```python
from build123d import *


with BuildPart() as part:
    # Sketch1 → Revolve1 (revolve)
    with BuildSketch(Plane(origin=(0, 0, 0), x_dir=(1, 0, 0), z_dir=(0, 1, 0))):
        with BuildLine():
            Line((-7.9375, -25.4), (-7.9375, 25.4))
            Line((-7.9375, 25.4), (-20.6375, 25.4))
            Line((-20.6375, 25.4), (-20.6375, -19.05))
            ThreePointArc((-20.6375, -19.05), (-54.768750138, -11.463041765), (-88.900000276, -19.05))
            Line((-88.900000276, -19.05), (-88.900000276, 126.999998896))
            Line((-88.900000276, 126.999998896), (-114.312969887, 126.999998896))
            ThreePointArc((-114.312969887, 126.999998896), (-190.5, 50.793515194), (-114.300000276, -25.4))
            Line((-114.300000276, -25.4), (-88.900000276, -25.4))
            ThreePointArc((-88.900000276, -25.4), (-54.768750138, -17.813041765), (-20.6375, -25.4))
            Line((-20.6375, -25.4), (-7.9375, -25.4))
        make_face()
    revolve(axis=Axis((0, 0, 25.4), (0, 0, -1)))


solid = part.part
```
The listing builds one solid part. Answer for the finished solid, in the listing's coordinates (mm). A direction names the side the tool comes from. Coordinates: 2 decimals unless noted, no trailing zeros. Loops run counter-clockwise (first coordinate to the right, second up) from the corner with the lowest first, then second, coordinate; pieces in that order, holes last. Notation, with made-up numbers: M 23,24 L 81,24 A13 cw 81,28 Z; hole C -2.75,9.25 d4. An arc over 180 degrees is marked long. Answer as a JSON object with one key per item and string values. Group by question number.
Item 1: Each of these flat-tipped pins is pushed along its axis until it touches: P1, Ø2, axis at x = 145, z = -49.5, coming from the +Y side; P2, Ø10, axis at x = -59.5, z = -18, coming from the +Y side; P3, Ø2, axis at y = 132, z = -39, coming from the -X side. Where does it stop, or does it pass through?
Item 2: Consider L1, parallel to Y at x = 0, z = -18; L2, parallel to Y at x = -74, z = -114; L3, parallel to X at y = 30.5, z = -47. Determine where each line is inside the solid, lowest interval first.
Item 3: Which of the six approach directions +Z, -Z, +X, -X, +Y, -Y give full straight-line access (tool end or side, diameter ignored) to faces 3 (the face through (4.474, -20.147, -2.864)), 4 (the face through (1.72, -7.75, -0.36))?
Item 4: Section A-A (z = -4.5) is taken. Write down the section's boundary in (x, y) (1 decimal).
Item 5: Determine the mould class of faces 1 (the face through (19.272, -86.786, -54.997)), 2 (the face through (0, -9, 25.4)) for opening direction Y: +Y half, -Y half, draft (parallel to the pull), parting line (faces both ways), or undercut.
Item 6: Section C-C (z = -112.5) is taken. Write down the section's boundary in (x, y).
Item 7: Section B-B (z = -71.5) is taken. Write down the section's boundary in (x, y), and give its area (3 significant figures).
Solved:
{
 "1": {"P1": "stops at y = 124.7", "P2": "stops at y = 176", "P3": "stops at x = -137.06"},
 "2": {"L1": "y = -183.08 to -88.9, -20.64 to -7.94, 7.94 to 20.64, 88.9 to 183.08", "L2": "y = -138.32 to -49.27, 49.27 to 138.32", "L3": "x = -187.95 to -83.5, 83.5 to 187.95"},
 "3": {"face 3": "-Z", "face 4": "+Z, -Z"},
 "4": {"outline": "C 0,0 d349.6; C 0,0 d41.3; hole C 0,0 d177.8; hole C 0,0 d15.9"},
 "5": {"face 1": "undercut", "face 2": "draft"},
 "6": {"outline": "C 0,0 d318.03; hole C 0,0 d177.8"},
 "7": {"outline": "C 0,0 d375.27; hole C 0,0 d177.8", "area": "85,800 mm2"}
}
